For this review, take the finished solid that the model builds, in its own axes (mm). Round coordinates to 2 decimals unless told otherwise and drop trailing zeros. Write each loop counter-clockwise with the first axis right and the second up, starting at its lowest first coordinate (ties: lowest second). Pieces come first, ordered by that corner, then holes. Notation, with made-up numbers: (34.25, -13.75) -> (83.25, -13.75) arc R14 ccw to (83.25, 2.25) -> close; hole circle Ø7 at (3, 65.25). An arc over 180 degrees is marked (long way). Answer in a Markdown table with one row per item. Add a question column.
```python
from build123d import *

# Parameters (mm, degrees)
SKETCH1_R           = 50
SKETCH1_R_2         = 1.9
BOSS_EXTRUDE1_DEPTH = 3.5
SKETCH2_R           = 4
CUT_EXTRUDE1_DEPTH  = 3.5
CIRPATTERN1_COUNT   = 16
CUT_EXTRUDE5_DEPTH  = 10
CIRPATTERN3_COUNT   = 3
SKETCH4_R           = 1.9
CUT_EXTRUDE6_DEPTH  = 3.5


with BuildPart() as part:
    # Sketch1 → Boss-Extrude1 (new body)
    with BuildSketch(Plane(origin=(0, 0, 0), x_dir=(1, 0, 0), z_dir=(0, 1, 0))):
        with Locations(Location((0, 0, 0), (0, 0, 270))):
            Circle(SKETCH1_R)
        with Locations(Location((0, 0, 0), (0, 0, 270))):
            Circle(SKETCH1_R_2, mode=Mode.SUBTRACT)
    extrude(amount=BOSS_EXTRUDE1_DEPTH)

    # Sketch2 → Cut-Extrude1 (cut)
    with BuildSketch(Plane(origin=(0, 3.5, 0), x_dir=(1, 0, 0), z_dir=(0, 1, 0))):
        with Locations(Location((0, 43, 0), (0, 0, 270))):
            Circle(SKETCH2_R)
    cut_extrude1 = extrude(amount=-CUT_EXTRUDE1_DEPTH, mode=Mode.SUBTRACT)

    # CirPattern1: Cut-Extrude1 ×16 about axis
    cirpattern1_axis = Axis((0, 0, 0), (0, 1, 0))
    for i in range(1, CIRPATTERN1_COUNT):
        add(cut_extrude1.rotate(cirpattern1_axis, i * 360 / CIRPATTERN1_COUNT), mode=Mode.SUBTRACT)

    # Sketch3 → Cut-Extrude5 (cut)
    with BuildSketch(Plane(origin=(0, 3.5, 0), x_dir=(1, 0, 0), z_dir=(0, 1, 0))):
        with BuildLine():
            ThreePointArc((7.794228634, 3.166666667), (11.088457268, -0.127561967), (15.588457268, -1.333333333))
            Line((15.588457268, -1.333333333), (29.634814361, -1.333333333))
            ThreePointArc((29.634814361, -1.333333333), (34.195516062, 0.767948929), (35.561777233, 5.6))
            ThreePointArc((35.561777233, 5.6), (23.0418607, 27.659946773), (-0.917016216, 35.988318678))
            ThreePointArc((-0.917016216, 35.988318678), (-5.998123181, 32.92383688), (-5.960332603, 26.990265565))
            Line((-5.960332603, 26.990265565), (0, 16.666666667))
            Line((0, 16.666666667), (7.794228634, 3.166666667))
        make_face()
    cut_extrude5 = extrude(amount=-CUT_EXTRUDE5_DEPTH, mode=Mode.SUBTRACT)

    # CirPattern3: Cut-Extrude5 ×3 about axis
    cirpattern3_axis = Axis((0, 0, 0), (0, 1, 0))
    for i in range(1, CIRPATTERN3_COUNT):
        add(cut_extrude5.rotate(cirpattern3_axis, i * 360 / CIRPATTERN3_COUNT), mode=Mode.SUBTRACT)

    # Sketch4 → Cut-Extrude6 (cut)
    with BuildSketch(Plane(origin=(0, 0, 0), x_dir=(1, 0, 0), z_dir=(0, 1, 0))):
        with Locations(Location((-1.230688491, 9.92398135, 0), (0, 0, 90))):
            Circle(SKETCH4_R)
        with Locations(Location((9.18308139, -3.899170456, 0), (0, 0, 90))):
            Circle(SKETCH4_R)
        with Locations(Location((-7.995004175, -6.006183819, 0), (0, 0, 90))):
            Circle(SKETCH4_R)
    extrude(amount=CUT_EXTRUDE6_DEPTH, mode=Mode.SUBTRACT)


solid = part.part
```
1. We need section D-D (z = 0). Write out the cut boundary in (x, y), plus the area to 3 significant figures.
2. We need section A-A (z = 30). Write out the cut boundary in (x, y).
3. We need section C-C (x = 22). Write out the cut boundary in (y, z).
4. Clearance check with flat-ended pins moving along their axes: pin 1 Ø2 at (y, z) = (0.5, -36.5) entering from +X; pin 2 Ø7 at (x, z) = (16.46, 39.73) entering from +Y; pin 3 Ø9 at (x, z) = (-39.73, -16.46) entering from +Y. State where each tip first meets the part, or that it passes through.
5. For L1, parallel to Z at x = -30, y = 0.3; L2, parallel to Z at x = 27, y = 0.75; L3, parallel to Z at x = -10, y = 1.7, list the stretches that pass through material, from the lowest coordinate up. Write a range as [from, to].
6. We need section B-B (x = -24). Write out the cut boundary in (y, z), plus the area to 3 significant figures.
Response:
| question | item | result |
|---|---|---|
| 1 | outline | (-50, 0) -> (-47, 0) -> (-47, 3.5) -> (-50, 3.5) -> close; (-39, 0) -> (-36, 0) -> (-36, 3.5) -> (-39, 3.5) -> close; (-9.62, 0) -> (-1.9, 0) -> (-1.9, 3.5) -> (-9.62, 3.5) -> close; (1.9, 0) -> (10.87, 0) -> (10.87, 3.5) -> (1.9, 3.5) -> close; (33.41, 0) -> (39, 0) -> (39, 3.5) -> (33.41, 3.5) -> close; (47, 0) -> (50, 0) -> (50, 3.5) -> (47, 3.5) -> close |
| 1 | area | 110 mm2 |
| 2 | outline | (-40, 0) -> (-34.38, 0) -> (-34.38, 3.5) -> (-40, 3.5) -> close; (-26.43, 0) -> (-16.43, 0) -> (-16.43, 3.5) -> (-26.43, 3.5) -> close; (19.9, 0) -> (26.43, 0) -> (26.43, 3.5) -> (19.9, 3.5) -> close; (34.38, 0) -> (40, 0) -> (40, 3.5) -> (34.38, 3.5) -> close |
| 3 | outline | (0, -44.9) -> (3.5, -44.9) -> (3.5, -28.5) -> (0, -28.5) -> close; (0, 1.33) -> (3.5, 1.33) -> (3.5, 8.33) -> (0, 8.33) -> close; (0, 28.5) -> (3.5, 28.5) -> (3.5, 44.9) -> (0, 44.9) -> close |
| 4 | pin 1 | x = 35.21 |
| 4 | pin 2 | through |
| 4 | pin 3 | y = 3.5 |
| 5 | L1 | [-40, -34.38], [-26.43, -19.9], [19.73, 26.43], [34.38, 40] |
| 5 | L2 | [-42.08, -32.5], [-28.31, -23.81], [1.33, 8.37], [23.81, 28.31], [32.5, 42.08] |
| 5 | L3 | [-48.99, -19.99], [0.65, 14.65], [34.58, 48.99] |
| 6 | outline | (0, -43.86) -> (3.5, -43.86) -> (3.5, -26.83) -> (0, -26.83) -> close; (0, 21.44) -> (3.5, 21.44) -> (3.5, 43.86) -> (0, 43.86) -> close |
| 6 | area | 138 mm2 |
